```python
from build123d import *

# Parameters (mm, degrees)
SKETCH1_W           = 12.8
SKETCH1_H           = 14.4
SKETCH1_R           = 2.25
BOSS_EXTRUDE1_DEPTH = 1.34
SKETCH2_R           = 2
BOSS_EXTRUDE2_DEPTH = 1.34
FILLET2_R           = 2
FILLET3_R           = 0.75
FILLET4_R           = 1.34


with BuildPart() as part:
    # Sketch1 → Boss-Extrude1 (new body)
    with BuildSketch(Plane(origin=(0, 0, 0), x_dir=(0, 0, -1), z_dir=(1, 0, 0))):
        with Locations((0, 7.2)):
            Rectangle(SKETCH1_W, SKETCH1_H)
        with Locations((0, 10.15)):
            Circle(SKETCH1_R, mode=Mode.SUBTRACT)
    extrude(amount=BOSS_EXTRUDE1_DEPTH)

    # Sketch2 → Boss-Extrude2 (add)
    with BuildSketch(Plane(origin=(0, 0, 0), x_dir=(1, 0, 0), z_dir=(0, 1, 0))):
        with BuildLine():
            Line((0, 6.4), (11.335489376, 6.4))
            ThreePointArc((11.335489376, 6.4), (15.5, 0), (11.335489376, -6.4))
            Line((11.335489376, -6.4), (0, -6.4))
            Line((0, -6.4), (0, 6.4))
        make_face()
        with Locations(Location((8, 0, 0), (0, 0, 270))):
            Circle(SKETCH2_R, mode=Mode.SUBTRACT)
    extrude(amount=BOSS_EXTRUDE2_DEPTH)

    # Fillet2
    fillet2_edges = [part.edges().sort_by_distance(p)[0] for p in [
        (0.67, 14.4, -6.4),
        (0.67, 14.4, 6.4),
    ]]
    fillet(fillet2_edges, radius=FILLET2_R)

    # Fillet3
    fillet3_edges = [part.edges().sort_by_distance(p)[0] for p in [
        (1.34, 1.34, 0),
    ]]
    fillet(fillet3_edges, radius=FILLET3_R)

    # Fillet4
    fillet4_edges = [part.edges().sort_by_distance(p)[0] for p in [
        (0, 0, 0),
    ]]
    fillet(fillet4_edges, radius=FILLET4_R)


solid = part.part
```
The listing builds one solid part. Answer for the finished solid, in the listing's coordinates (mm). A direction names the side the tool comes from. Coordinates: 2 decimals unless noted, no trailing zeros. Loops run counter-clockwise (first coordinate to the right, second up) from the corner with the lowest first, then second, coordinate; pieces in that order, holes last. Notation, with made-up numbers: M 74,49 L 105,49 A20 ccw 105,54 Z; hole C -27.5,32.5 d9. An arc over 180 degrees is marked long. Answer as a JSON object with one key per item and string values. Group by question number.
Item 1: Which of the six approach directions +Z, -Z, +X, -X, +Y, -Y give full straight-line access (tool end or side, diameter ignored) to faces 4 (the face through (10.4, 1.34, -0.1)), 5 (the face through (0.68, 13.8, 5.83))?
Item 2: Each of these flat-tipped pins is pushed along its axis until it touches: P1, Ø1.5, axis at y = 10.5, z = 2, coming from the +X side; P2, Ø6.5, axis at x = 8, z = 0, coming from the -Y side; P3, Ø6.5, axis at x = 6.5, z = 1.5, coming from the +Y side. Where does it stop, or does it pass through?
Item 3: Section C-C (x = 8) is taken. Write down the section's boundary in (y, z).
Item 4: Determine the mould class of faces 1 (the face through (0, 7, 0)), 2 (the face through (0.68, 13.8, -5.83)), 3 (the face through (10, 1, 0)) for opening direction X: +X half, -X half, draft (parallel to the pull), parting line (faces both ways), or undercut.
Item 5: Section D-D (z = -3) is taken. Write down the section's boundary in (x, y).
Item 6: Consider L1, parallel to Y at x = 12.75, z = -2; L2, parallel to X at y = 0.45, z = 0. Determine where each line is inside the solid, lowest interval first.
Item 7: Section A-A (y = 11.5) is taken. Write down the section's boundary in (x, z), and give its area (3 significant figures).
Item 8: Section B-B (z = 0) is taken. Write down the section's boundary in (x, y).
Solved:
{
 "1": {"face 4": "+Z, -Z, +X, +Y", "face 5": "+Z, +X, -X, +Y"},
 "2": {"P1": "stops at x = 1.34", "P2": "stops at y = 0", "P3": "stops at y = 1.34"},
 "3": {"outline": "M 0,-6.4 L 1.34,-6.4 L 1.34,-2 L 0,-2 Z; M 0,2 L 1.34,2 L 1.34,6.4 L 0,6.4 Z"},
 "4": {"face 1": "-X half", "face 2": "draft", "face 3": "undercut"},
 "5": {"outline": "M 0,1.34 A1.34 ccw 1.34,0 L 14.82,0 L 14.82,1.34 L 2.09,1.34 A0.75 cw 1.34,2.09 L 1.34,14.4 L 0,14.4 Z"},
 "6": {"L1": "y = 0 to 1.34", "L2": "x = 0.34 to 6, 10 to 15.5"},
 "7": {"outline": "M 0,-6.4 L 1.34,-6.4 L 1.34,-1.8 L 0,-1.8 Z; M 0,1.8 L 1.34,1.8 L 1.34,6.4 L 0,6.4 Z", "area": "12.3 mm2"},
 "8": {"outline": "M 0,1.34 A1.34 ccw 1.34,0 L 6,0 L 6,1.34 L 2.09,1.34 A0.75 cw 1.34,2.09 L 1.34,7.9 L 0,7.9 Z; M 0,12.4 L 1.34,12.4 L 1.34,14.4 L 0,14.4 Z; M 10,0 L 15.5,0 L 15.5,1.34 L 10,1.34 Z"}
}
